The listing builds one solid part. Answer for the finished solid, in the listing's coordinates (mm). A direction names the side the tool comes from. Give positions to 0.01 mm unless a question says otherwise; leave off trailing zeros. Order: outer loops, then holes, each group sorted by start corner. A loop starts at its lowest first (then second) coordinate and runs counter-clockwise, first axis right, second up. Notation, with made-up numbers: (39, 28) - (73, 28) arc R22 cw to (73, 44) - close; hole circle Ø3 at (15.25, 44). An arc over 180 degrees is marked (long way). Answer in a Markdown table with one row per item.
from build123d import *

# Parameters (mm, degrees)
SKETCH1_W            = 150
SKETCH1_H            = 130
BOSS_EXTRUDE1_DEPTH  = 2.5
SKETCH2_W            = 150
SKETCH2_H            = 130
BOSS_EXTRUDE2_DEPTH  = 2
SKETCH3_W            = 2.5
SKETCH3_H            = 16.780539685
BOSS_EXTRUDE3_DEPTH  = 12
SKETCH4_W            = 6.999579775
SKETCH4_H            = 4.214800725
SKETCH4_W_2          = 6.547993983
SKETCH4_H_2          = 4.177168575
CUT_EXTRUDE1_DEPTH   = 12
SKETCH5_W            = 13.520958653
SKETCH5_H            = 1.542676049
SKETCH5_H_2          = 1.182146985
BOSS_EXTRUDE4_DEPTH  = 12.5
SKETCH6_W            = 16.86645729
SKETCH6_H            = 7.123900825
BOSS_EXTRUDE5_DEPTH  = 2.5
SKETCH7_W            = 13.933318375
SKETCH7_H            = 1.459493224
SKETCH7_H_2          = 2.069451468
BOSS_EXTRUDE6_DEPTH  = 10.5
SKETCH8_W            = 1.465633043
SKETCH8_H            = 7.120231944
SKETCH8_W_2          = 2.837736244
SKETCH8_H_2          = 7.249129709
BOSS_EXTRUDE8_DEPTH  = 10.5
SKETCH9_W            = 11.026219754
SKETCH9_H            = 2.333193258
SKETCH9_W_2          = 2.290453933
SKETCH9_H_2          = 3.041515947
SKETCH9_W_3          = 1.716125118
SKETCH9_H_3          = 6.956645693
BOSS_EXTRUDE9_DEPTH  = 8.5
SKETCH10_W           = 64.150572822
SKETCH10_H           = 1.749214845
CUT_EXTRUDE2_DEPTH   = 22
SKETCH11_R           = 4
SKETCH11_R_2         = 4.5
BOSS_EXTRUDE10_DEPTH = 2.5
SKETCH12_R           = 1.35
CUT_EXTRUDE3_DEPTH   = 5
SKETCH13_R           = 1.6
CUT_EXTRUDE4_DEPTH   = 9
CHAMFER1_SIZE        = 1.5
FILLET1_R            = 2
SKETCH14_W           = 2.326153497
SKETCH14_H           = 19.505362719
BOSS_EXTRUDE11_DEPTH = 11
SKETCH15_W           = 116.835015105
SKETCH15_H           = 2.5
BOSS_EXTRUDE12_DEPTH = 37
SKETCH16_W           = 2.915269742
SKETCH16_H           = 2.460041161
BOSS_EXTRUDE13_DEPTH = 33


with BuildPart() as part:
    # Sketch1 → Boss-Extrude1 (new body)
    with BuildSketch(Plane(origin=(0, 0, 0), x_dir=(1, 0, 0), z_dir=(0, 1, 0))):
        with Locations((10.867486339, -10.655737705)):
            Rectangle(SKETCH1_W, SKETCH1_H)
    extrude(amount=BOSS_EXTRUDE1_DEPTH)

    # Sketch2 → Boss-Extrude2 (add)
    with BuildSketch(Plane.XZ):
        with Locations((10.867486339, 10.655737705)):
            Rectangle(SKETCH2_W, SKETCH2_H)
    extrude(amount=BOSS_EXTRUDE2_DEPTH)

    # Sketch3 → Boss-Extrude3 (add)
    with BuildSketch(Plane(origin=(0, 2.5, 0), x_dir=(1, 0, 0), z_dir=(0, 1, 0))):
        with Locations((-49.882513661, -50.670528215)):
            Rectangle(SKETCH3_W, SKETCH3_H)
    extrude(amount=BOSS_EXTRUDE3_DEPTH)

    # Sketch4 → Cut-Extrude1 (cut)
    with BuildSketch(Plane(origin=(0, 14.5, 0), x_dir=(1, 0, 0), z_dir=(0, 1, 0))):
        with Locations((-49.30282547, -47.109594286)):
            Rectangle(SKETCH4_W, SKETCH4_H)
        with Locations((-49.077032574, -54.692472376)):
            Rectangle(SKETCH4_W_2, SKETCH4_H_2)
    extrude(amount=-CUT_EXTRUDE1_DEPTH, mode=Mode.SUBTRACT)

    # Sketch5 → Boss-Extrude4 (add)
    with BuildSketch(Plane(origin=(0, 2.5, 0), x_dir=(1, 0, 0), z_dir=(0, 1, 0))):
        with Locations((-55.392992988, -59.832136082)):
            Rectangle(SKETCH5_W, SKETCH5_H)
        with Locations((-55.392992988, -41.68918488)):
            Rectangle(SKETCH5_W, SKETCH5_H_2)
    extrude(amount=BOSS_EXTRUDE4_DEPTH)

    # Sketch6 → Boss-Extrude5 (add)
    with BuildSketch(Plane(origin=(0, 2.5, 0), x_dir=(1, 0, 0), z_dir=(0, 1, 0))):
        with Locations((-50.314672673, -69.866817827)):
            Rectangle(SKETCH6_W, SKETCH6_H)
    extrude(amount=BOSS_EXTRUDE5_DEPTH)

    # Sketch7 → Boss-Extrude6 (add)
    with BuildSketch(Plane(origin=(0, 2.5, 0), x_dir=(1, 0, 0), z_dir=(0, 1, 0))):
        with Locations((-55.033530113, -26.576664837)):
            Rectangle(SKETCH7_W, SKETCH7_H)
        with Locations((-55.033530113, -36.325889274)):
            Rectangle(SKETCH7_W, SKETCH7_H_2)
    extrude(amount=BOSS_EXTRUDE6_DEPTH)

    # Sketch8 → Boss-Extrude8 (add)
    with BuildSketch(Plane(origin=(0, 2.5, 0), x_dir=(1, 0, 0), z_dir=(0, 1, 0))):
        with Locations((-40.946126135, -62.470830958)):
            Rectangle(SKETCH8_W, SKETCH8_H)
        with Locations((-30.762507723, -62.68030256)):
            Rectangle(SKETCH8_W_2, SKETCH8_H_2)
    extrude(amount=BOSS_EXTRUDE8_DEPTH)

    # Sketch9 → Boss-Extrude9 (add)
    with BuildSketch(Plane(origin=(0, 2.5, 0), x_dir=(1, 0, 0), z_dir=(0, 1, 0))):
        with Locations((-22.326370107, -59.157602986)):
            Rectangle(SKETCH9_W, SKETCH9_H)
        with Locations((-15.699052952, -71.779845012)):
            Rectangle(SKETCH9_W_2, SKETCH9_H_2)
        with Locations((-28.697542543, -70.271634632)):
            Rectangle(SKETCH9_W_3, SKETCH9_H_3)
    extrude(amount=BOSS_EXTRUDE9_DEPTH)

    # Sketch10 → Cut-Extrude2 (cut)
    with BuildSketch(Plane(origin=(0, 2.5, 0), x_dir=(1, 0, 0), z_dir=(0, 1, 0))):
        with Locations((-28.662922823, -73.523219452)):
            Rectangle(SKETCH10_W, SKETCH10_H)
    extrude(amount=CUT_EXTRUDE2_DEPTH, mode=Mode.SUBTRACT)

    # Sketch11 → Boss-Extrude10 (add)
    with BuildSketch(Plane(origin=(0, 2.5, 0), x_dir=(1, 0, 0), z_dir=(0, 1, 0))):
        with Locations(Location((61.867486339, -2.855737705, 0), (0, 0, 270))):
            Circle(SKETCH11_R)
        with Locations(Location((76.867486339, 28.044262295, 0), (0, 0, 270))):
            Circle(SKETCH11_R)
        with Locations(Location((51.867486339, 43.344262295, 0), (0, 0, 270))):
            Circle(SKETCH11_R_2)
        with Locations(Location((51.867486339, -12.655737705, 0), (0, 0, 270))):
            Circle(SKETCH11_R)
        with Locations(Location((-53.132513661, -12.655737705, 0), (0, 0, 270))):
            Circle(SKETCH11_R)
        with Locations(Location((-53.132513661, 43.344262295, 0), (0, 0, 270))):
            Circle(SKETCH11_R)
    extrude(amount=BOSS_EXTRUDE10_DEPTH)

    # Sketch12 → Cut-Extrude3 (cut)
    with BuildSketch(Plane(origin=(0, 5, 0), x_dir=(1, 0, 0), z_dir=(0, 1, 0))):
        with Locations(Location((-53.208473164, -12.731303325, 0), (0, 0, 270))):
            Circle(SKETCH12_R)
        with Locations(Location((-53.132513661, 43.344262295, 0), (0, 0, 270))):
            Circle(SKETCH12_R)
        with Locations(Location((51.867486339, 43.344262295, 0), (0, 0, 270))):
            Circle(SKETCH12_R)
        with Locations(Location((51.867486339, -12.655737705, 0), (0, 0, 270))):
            Circle(SKETCH12_R)
        with Locations(Location((61.867486339, -2.855737705, 0), (0, 0, 270))):
            Circle(SKETCH12_R)
        with Locations(Location((76.867486339, 28.044262295, 0), (0, 0, 270))):
            Circle(SKETCH12_R)
    extrude(amount=-CUT_EXTRUDE3_DEPTH, mode=Mode.SUBTRACT)

    # Sketch13 → Cut-Extrude4 (cut)
    with BuildSketch(Plane.XZ.offset(2)):
        with Locations(Location((-61.332513661, 72.655737705, 0), (0, 0, 270))):
            Circle(SKETCH13_R)
        with Locations(Location((3.254378963, 71.655737705, 0), (0, 0, 270))):
            Circle(SKETCH13_R)
        with Locations(Location((82.867486339, 72.655737705, 0), (0, 0, 270))):
            Circle(SKETCH13_R)
        with Locations(Location((82.367486339, -50.844262295, 0), (0, 0, 270))):
            Circle(SKETCH13_R)
        with Locations(Location((-60.632513661, -50.844262295, 0), (0, 0, 270))):
            Circle(SKETCH13_R)
        with Locations(Location((7.222931356, -51.344262295, 0), (0, 0, 270))):
            Circle(SKETCH13_R)
        with Locations(Location((-60.132513661, 21.175451705, 0), (0, 0, 270))):
            Circle(SKETCH13_R)
        with Locations(Location((82.055017687, 12.739317464, 0), (0, 0, 270))):
            Circle(SKETCH13_R)
    extrude(amount=-CUT_EXTRUDE4_DEPTH, mode=Mode.SUBTRACT)

    # Chamfer1
    # the kernel refuses this chamfer: 1.5 mm, written as the material it takes off along each edge
    with BuildSketch(Plane(origin=(3.254378963, -2, 71.655737705), x_dir=(0, 0, -1), z_dir=(-1, 0, 0))) as chamfer1_piece_1:
        Polygon((1.6 + CHAMFER1_SIZE, 0), (1.6, -CHAMFER1_SIZE), (1.6, 0), align=None)
    revolve(axis=Axis((3.254378963, -2, 71.655737705), (0, -1, 0)), mode=Mode.SUBTRACT)
    with BuildSketch(Plane(origin=(82.867486339, -2, 72.655737705), x_dir=(0, 0, -1), z_dir=(-1, 0, 0))) as chamfer1_piece_2:
        Polygon((1.6 + CHAMFER1_SIZE, 0), (1.6, -CHAMFER1_SIZE), (1.6, 0), align=None)
    revolve(axis=Axis((82.867486339, -2, 72.655737705), (0, -1, 0)), mode=Mode.SUBTRACT)
    with BuildSketch(Plane(origin=(82.367486339, -2, -50.844262295), x_dir=(0, 0, -1), z_dir=(-1, 0, 0))) as chamfer1_piece_3:
        Polygon((1.6 + CHAMFER1_SIZE, 0), (1.6, -CHAMFER1_SIZE), (1.6, 0), align=None)
    revolve(axis=Axis((82.367486339, -2, -50.844262295), (0, -1, 0)), mode=Mode.SUBTRACT)
    with BuildSketch(Plane(origin=(-60.632513661, -2, -50.844262295), x_dir=(0, 0, -1), z_dir=(-1, 0, 0))) as chamfer1_piece_4:
        Polygon((1.6 + CHAMFER1_SIZE, 0), (1.6, -CHAMFER1_SIZE), (1.6, 0), align=None)
    revolve(axis=Axis((-60.632513661, -2, -50.844262295), (0, -1, 0)), mode=Mode.SUBTRACT)
    with BuildSketch(Plane(origin=(7.222931356, -2, -51.344262295), x_dir=(0, 0, -1), z_dir=(-1, 0, 0))) as chamfer1_piece_5:
        Polygon((1.6 + CHAMFER1_SIZE, 0), (1.6, -CHAMFER1_SIZE), (1.6, 0), align=None)
    revolve(axis=Axis((7.222931356, -2, -51.344262295), (0, -1, 0)), mode=Mode.SUBTRACT)
    with BuildSketch(Plane(origin=(-60.132513661, -2, 21.175451705), x_dir=(0, 0, -1), z_dir=(-1, 0, 0))) as chamfer1_piece_6:
        Polygon((1.6 + CHAMFER1_SIZE, 0), (1.6, -CHAMFER1_SIZE), (1.6, 0), align=None)
    revolve(axis=Axis((-60.132513661, -2, 21.175451705), (0, -1, 0)), mode=Mode.SUBTRACT)
    with BuildSketch(Plane(origin=(82.055017687, -2, 12.739317464), x_dir=(0, 0, -1), z_dir=(-1, 0, 0))) as chamfer1_piece_7:
        Polygon((1.6 + CHAMFER1_SIZE, 0), (1.6, -CHAMFER1_SIZE), (1.6, 0), align=None)
    revolve(axis=Axis((82.055017687, -2, 12.739317464), (0, -1, 0)), mode=Mode.SUBTRACT)
    with BuildSketch(Plane(origin=(-61.332513661, -2, 72.655737705), x_dir=(0, 0, -1), z_dir=(-1, 0, 0))) as chamfer1_piece_8:
        Polygon((1.6 + CHAMFER1_SIZE, 0), (1.6, -CHAMFER1_SIZE), (1.6, 0), align=None)
    revolve(axis=Axis((-61.332513661, -2, 72.655737705), (0, -1, 0)), mode=Mode.SUBTRACT)

    # Fillet1
    # the kernel refuses this fillet: 2 mm, written as the material it takes off along each edge
    with BuildSketch(Plane(origin=(-64.132513661, -7, -54.344262295), x_dir=(1, 0, 0), z_dir=(0, 1, 0)), Plane(origin=(85.867486339, 7.5, -54.344262295), x_dir=(-1, 0, 0), z_dir=(0, -1, 0)), Plane(origin=(85.867486339, 7.5, 75.655737705), x_dir=(0, 0, -1), z_dir=(0, -1, 0)), Plane(origin=(-64.132513661, -7, 75.655737705), x_dir=(0, 0, -1), z_dir=(0, 1, 0))) as fillet1_piece_1:
        with BuildLine():
            CenterArc((FILLET1_R, -FILLET1_R), FILLET1_R, 90, 90)
            Line((0, -FILLET1_R), (0, 0))
            Line((0, 0), (FILLET1_R, 0))
        make_face()
    extrude(amount=14.5, mode=Mode.SUBTRACT)

    # Sketch14 → Boss-Extrude11 (add)
    with BuildSketch(Plane(origin=(0, 14.5, 0), x_dir=(1, 0, 0), z_dir=(0, 1, 0))):
        with Locations((-49.79559041, -50.850792747)):
            Rectangle(SKETCH14_W, SKETCH14_H)
    extrude(amount=BOSS_EXTRUDE11_DEPTH)

    # Sketch15 → Boss-Extrude12 (add)
    with BuildSketch(Plane(origin=(0, 2.5, 0), x_dir=(1, 0, 0), z_dir=(0, 1, 0))):
        with Locations((-0.676686853, -19.412678434)):
            Rectangle(SKETCH15_W, SKETCH15_H)
    extrude(amount=BOSS_EXTRUDE12_DEPTH)

    # Sketch16 → Boss-Extrude13 (add)
    with BuildSketch(Plane(origin=(0, 39.5, 0), x_dir=(1, 0, 0), z_dir=(0, 1, 0))):
        with Locations((-60.551829276, -19.392699014)):
            Rectangle(SKETCH16_W, SKETCH16_H)
    extrude(amount=-BOSS_EXTRUDE13_DEPTH)


solid = part.part
Item 1: Each of these flat-tipped pins is pushed along its axis until it touches: P1, Ø0.8, axis at x = 52.5, z = -43, coming from the +Y side; P2, Ø2.5, axis at x = -60.5, y = 15.5, coming from the +Z side; P3, Ø2, axis at x = -61, z = 19, coming from the -Y side; P4, Ø1.2, axis at x = -50, z = 53.5, coming from the +Y side. Where does it stop, or does it pass through?
Answer block:
| item | result |
|---|---|
| P1 | y = 0 |
| P2 | z = 60.6 |
| P3 | y = -2 |
| P4 | y = 25.5 |
Item 2: Find section C-C on x = -23. Write down the section's boundary in (y, z).
Answer block:
| item | result |
|---|---|
| outline | (-2, -54.34) - (2.5, -54.34) - (2.5, 18.16) - (39.5, 18.16) - (39.5, 20.66) - (2.5, 20.66) - (2.5, 57.99) - (11, 57.99) - (11, 60.32) - (2.5, 60.32) - (2.5, 75.66) - (-2, 75.66) - close |
Item 3: Find section B-B on x = -44.5. Write down the section's boundary in (y, z), then the cut area to 3 significant figures.
Answer block:
| item | result |
|---|---|
| outline | (-2, -54.34) - (2.5, -54.34) - (2.5, 18.16) - (39.5, 18.16) - (39.5, 20.66) - (2.5, 20.66) - (2.5, 66.3) - (5, 66.3) - (5, 72.65) - (2.5, 72.65) - (2.5, 75.66) - (-2, 75.66) - close |
| area | 693 mm² |
Item 4: Consider line 1 (Y direction, x = -11.5, z = 64.5); line 2 (Z direction, x = 15.5, y = 19.5); line 3 (X direction, y = 24.5, z = 51.5). Determine where each line is inside the solid, lowest interval first.
Answer block:
| item | result |
|---|---|
| line 1 | -2 to 2.5 |
| line 2 | 18.16 to 20.66 |
| line 3 | -50.96 to -48.63 |
Item 5: Which of the six approach directions +Z, -Z, +X, -X, +Y, -Y give full straight-line access (tool end or side, diameter ignored) to faces 1 (the face through (-29.556, 7, 70)), 2 (the face through (-22, 7, 60.324)), 3 (the face through (-55, 8, 35.291))?
Answer block:
| item | result |
|---|---|
| face 1 | +Z, +Y |
| face 2 | +Z, +X, +Y |
| face 3 | +X, -X, +Y |
Item 6: Determine the mould class of faces 4 (the face through (10, 0, 75.656)), 5 (the face through (62, 5, 5)), 6 (the face through (52.07, 3.73, -47.84)), 7 (the face through (-55, 9, 41.098)) for opening direction Z: pulls with the +Z half, pulls with the -Z half, needs draft (parallel to the pull), parting line crosses it, or undercut.
Answer block:
| item | result |
|---|---|
| face 4 | pulls with the +Z half |
| face 5 | needs draft |
| face 6 | undercut |
| face 7 | undercut |
